Can you work these out from the model? Positions are in its coordinate system, mm. Face numbers are marked on the shaded views. Give positions to 0.01 mm unless a question says otherwise; leave off trailing zeros. Write each loop counter-clockwise with the first axis right and the second up, starting at its lowest first coordinate (ties: lowest second). Pieces come first, ordered by that corner, then holes.
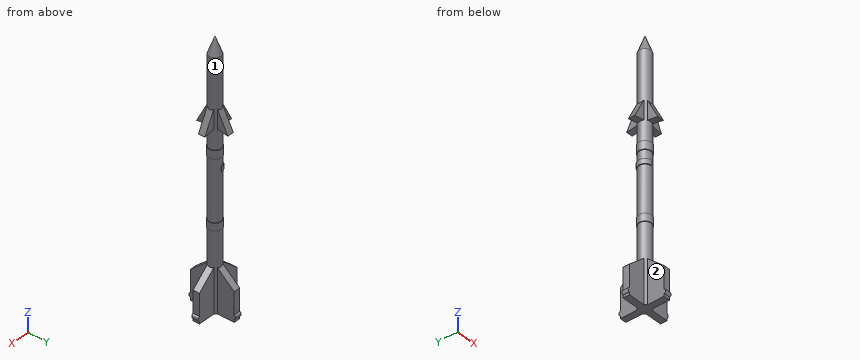
```python
from build123d import *

# Parameters (mm, degrees)
F3_DEPTH      = 0.3
F4_COUNT      = 4
F5_W          = 0.625
F5_H          = 0.4513888889
F6_ANGLE_BACK = 90
F6_ANGLE      = 180


with BuildPart() as f1:
    # F0 (on Front) → F1 (revolve)
    with BuildSketch(Plane.XZ):
        Polygon((0, 24.1666666667), (0, 0), (0.5555555556, 0), (0.5555555556, 7.3611111111), (0.6076388889, 7.3611111111), (0.6076388889, 8.0555555556), (0.5555555556, 8.0555555556), (0.5555555556, 13.7152777778), (0.6076388889, 13.7152777778), (0.6076388889, 14.4791666667), (0.5555555556, 14.4791666667), (0.5555555556, 22.6388888889), align=None)
    revolve(axis=Axis((0, 0, 12.0833333333), (0, 0, -1)))

    # F2 (on Front) → F3 (join, symmetric)
    with BuildSketch(Plane.XZ):
        with BuildLine():
            Line((0, 0), (2.0486111111, 0))
            Line((2.0486111111, 0), (2.0486111111, 0.2430555556))
            ThreePointArc((2.0486111111, 0.2430555556), (2.1875, 0.4513888889), (2.0486111111, 0.6597222222))
            Line((2.0486111111, 0.6597222222), (2.0486111111, 2.7083333333))
            Line((2.0486111111, 2.7083333333), (0.4, 4.165245478))
            Line((0.4, 4.165245478), (0.4, 16.3433760684))
            Line((0.4, 16.3433760684), (1.4583333333, 16.1805555556))
            Line((1.4583333333, 16.1805555556), (0, 19.0411324786))
            Line((0, 19.0411324786), (0, 0))
        make_face()
    extrude(amount=F3_DEPTH, both=True)

    # F4: F1 ×4 about axis
    f4_axis = Axis((0, 0, 8.0555555556), (0, 0, 1))


with BuildPart() as f1_1:
    add(f1.part)
    for i in range(1, F4_COUNT):
        add(f1.part.rotate(f4_axis, i * 360 / F4_COUNT))

    # F5 (on Front) → F6 (revolve)
    with BuildSketch(Plane.XZ, mode=Mode.PRIVATE) as f6_sk:
        with Locations((-0.3125, 12.65625)):
            Rectangle(F5_W, F5_H)
    revolve(f6_sk.sketch.rotate(Axis((0, 0, 8.0555555556), (0, 0, 1)), -F6_ANGLE_BACK), axis=Axis((0, 0, 8.0555555556), (0, 0, 1)), revolution_arc=F6_ANGLE)


solid = f1_1.part
```
1) For pin 1 Ø2 at (x, z) = (0, 13) entering from +Y (3 decimals); pin 2 Ø1.4 at (y, z) = (-1.5, 2) entering from +X; pin 3 Ø1.5 at (y, z) = (0.5, 19.5) entering from +X, each with a flat end and sliding along its axis, tell me the tip position at first contact or that it passes through.
Values follow:
pin 1: stops at y = 0.625
pin 2: stops at x = 0.3
pin 3: stops at x = 0.56
2) Suppose I cut it at C-C on z = 7.75. Write out the boundary of the cut face in (x, y).
Values follow:
outline: circle Ø1.22 at (0, 0)
3) If we mould it in two halves opening along Z, with no side actions, what happens to the marked faces 1 and 2? For each: +Z half, -Z half, draft (parallel to the pull), parting line (faces both ways), or undercut.
Values follow:
face 1: undercut
face 2: draft
4) Suppose I cut it at A-A on x = 1.15. Write out the boundary of the cut face in (y, z), plus the area to 3 significant figures.
Values follow:
outline: (-0.3, 0) - (0.3, 0) - (0.3, 3.5) - (-0.3, 3.5) - close; (-0.3, 16.23) - (0.3, 16.23) - (0.3, 16.79) - (-0.3, 16.79) - close
area: 2.44 mm2
5) Please list where these lines run through material, in increasing order: L1, parallel to Y at x = -1.7, z = 1; L2, parallel to X at y = 0.05, z = 13; L3, parallel to Z at x = -0.85, y = -0.2.
Values follow:
L1: y = -0.3 to 0.3
L2: x = -0.55 to 0.55
L3: z = 0 to 3.77, 16.27 to 17.37
6) Suppose I cut it at B-B on z = 4.75. Write out the boundary of the cut face in (x, y).
Values follow:
outline: circle Ø1.11 at (0, 0)
